```python
from build123d import *

# Parameters (mm, degrees)
BOSS_EXTRUDE1_DEPTH = 15
BOSS_EXTRUDE2_DEPTH = 20
SKETCH3_R           = 2.25
CUT_EXTRUDE1_DEPTH  = 15


with BuildPart() as part:
    # Sketch1 → Boss-Extrude1 (new, symmetric)
    with BuildSketch(Plane(origin=(0, 0, 0), x_dir=(1, 0, 0), z_dir=(0, 1, 0))):
        with BuildLine():
            Line((0, 0), (-27.5, 0))
            Line((-27.5, 0), (-22.5, -5))
            Line((-22.5, -5), (-44.5, -5))
            Line((-44.5, -5), (-44.5, 10))
            Line((-44.5, 10), (-35, 10))
            Line((-35, 10), (-35, 20))
            Line((-35, 20), (-25, 20))
            ThreePointArc((-25, 20), (-17.5, 12.5), (-10, 20))
            Line((-10, 20), (10, 20))
            ThreePointArc((10, 20), (17.5, 12.5), (25, 20))
            Line((25, 20), (35, 20))
            Line((35, 20), (35, 10))
            Line((35, 10), (44.5, 10))
            Line((44.5, 10), (44.5, -5))
            Line((44.5, -5), (22.5, -5))
            Line((22.5, -5), (27.5, 0))
            Line((27.5, 0), (0, 0))
        make_face()
    extrude(amount=BOSS_EXTRUDE1_DEPTH, both=True)

    # Sketch2 → Boss-Extrude2 (add, symmetric)
    with BuildSketch(Plane(origin=(0, 0, 0), x_dir=(1, 0, 0), z_dir=(0, 1, 0))):
        with BuildLine():
            Line((-30, 20), (-25, 20))
            ThreePointArc((-25, 20), (-17.5, 12.5), (-10, 20))
            Line((-10, 20), (5, 20))
            Line((5, 20), (10, 20))
            ThreePointArc((10, 20), (17.5, 12.5), (25, 20))
            Line((25, 20), (30, 20))
            ThreePointArc((30, 20), (26.338834765, 11.161165235), (17.5, 7.5))
            Line((17.5, 7.5), (7.664635512, 7.5))
            Line((7.664635512, 7.5), (7.664635512, 0))
            Line((7.664635512, 0), (-7.335364488, 0))
            Line((-7.335364488, 0), (-7.335364488, 7.5))
            Line((-7.335364488, 7.5), (-17.5, 7.5))
            ThreePointArc((-17.5, 7.5), (-26.338834765, 11.161165235), (-30, 20))
        make_face()
    extrude(amount=BOSS_EXTRUDE2_DEPTH, both=True)

    # Sketch3 → Cut-Extrude1 (cut)
    with BuildSketch(Plane(origin=(0, 0, -20), x_dir=(-1, 0, 0), z_dir=(0, 0, -1))):
        with Locations((0, 15)):
            Circle(SKETCH3_R)
        with Locations((-30, 7.5)):
            Circle(SKETCH3_R)
        with Locations((-30, -7.5)):
            Circle(SKETCH3_R)
        with Locations(Location((30, -7.5, 0), (0, 0, 180))):
            Circle(SKETCH3_R)
        with Locations(Location((30, 7.5, 0), (0, 0, 180))):
            Circle(SKETCH3_R)
        with Locations(Location((0, -15, 0), (0, 0, 180))):
            Circle(SKETCH3_R)
    extrude(amount=-CUT_EXTRUDE1_DEPTH, mode=Mode.SUBTRACT)


solid = part.part
```
Input: part model. Units: mm. Frame: model coordinates. A direction names the side the tool comes from. Give positions to 0.01 mm unless a question says otherwise; leave off trailing zeros. Order: outer loops, then holes, each group sorted by start corner. A loop starts at its lowest first (then second) coordinate and runs counter-clockwise, first axis right, second up. Notation, with made-up numbers: M 16.25,-39 L 58.25,-39 A30 ccw 58.25,-15 Z; hole C 69.5,-1.75 d4. An arc over 180 degrees is marked long. Return JSON: item names as keys, results as strings.
1) Section query D-D on z = -8.5. Output: boundary loops of the cut face in (x, y), and give its area (3 significant figures).
Taken from the geometry:
{"outline": "M -44.5,-15 L -22.4,-15 L -22.4,-20 L 22.4,-20 L 22.4,-15 L 44.5,-15 L 44.5,15 L 22.4,15 L 22.4,20 L -22.4,20 L -22.4,15 L -44.5,15 Z; hole C -30,-7.5 d4.5; hole C -30,7.5 d4.5; hole C 0,-15 d4.5; hole C 0,15 d4.5; hole C 30,-7.5 d4.5; hole C 30,7.5 d4.5", "area": "3,020 mm2"}
2) Access query for faces 1 (the face through (-35, 0, -15)), 2 (the face through (-12, -17, -7.5)), 3 (the face through (0, 15, -5)), 4 (the face through (13, 18, -7.5)). Directions: +Z, -Z, +X, -X, +Y, -Y. A direction counts if a zero-diameter tool reaches every point of the face in a straight line with its end or side. Return the directions, or none.
Taken from the geometry:
{"face 1": "-Z, -X, +Y, -Y", "face 2": "+Z, -X, -Y", "face 3": "-Z", "face 4": "+Z, +X, +Y"}
3) Section query B-B on z = -3.75. Output: boundary loops of the cut face in (x, y), and give its area (3 significant figures).
Taken from the geometry:
{"outline": "M -44.5,-15 L -7.34,-15 L -7.34,-20 L 7.66,-20 L 7.66,-15 L 44.5,-15 L 44.5,15 L 7.66,15 L 7.66,20 L -7.34,20 L -7.34,15 L -44.5,15 Z", "area": "2,820 mm2"}
4) Line query: L1, parallel to Y at x = -30, z = -9.5; L2, parallel to Y at x = 35, z = -3; L3, parallel to Z at x = -27, y = -11. Output: solid intervals per line, ascending. Write a range as [from, to].
Taken from the geometry:
{"L1": "y = [-15, -9.75], [-5.25, 5.25], [9.75, 15]", "L2": "y = [-15, 15]", "L3": "z = [-20, 0], [0.5, 5]"}
5) Section query A-A on y = 7.5. Output: boundary loops of the cut face in (x, z), and give its area (3 significant figures).
Taken from the geometry:
{"outline": "M -44.5,-10 L -35,-10 L -35,-20 L -32.25,-20 L -32.25,-5 L -27.75,-5 L -27.75,-20 L -25,-20 A7.5 cw -10,-20 L 10,-20 A7.5 cw 25,-20 L 27.75,-20 L 27.75,-5 L 32.25,-5 L 32.25,-20 L 35,-20 L 35,-10 L 44.5,-10 L 44.5,5 L 22.5,5 L 27.5,0 L -27.5,0 L -22.5,5 L -44.5,5 Z", "area": "1,470 mm2"}
6) Section query C-C on x = 38. Output: boundary loops of the cut face in (y, z), and give its area (3 significant figures).
Taken from the geometry:
{"outline": "M -15,-10 L 15,-10 L 15,5 L -15,5 Z", "area": "450 mm2"}
7) Mould query, pull axis Y, two halves, no side actions, for faces 5 (the face through (-12, 18, -7.5)), 6 (the face through (30, -15, -5)), 7 (the face through (30, 15, -5)), 8 (the face through (0, -15, -5)). Classes: released by +Y, released by -Y, zero draft, split by the parting line, or undercut.
Taken from the geometry:
{"face 5": "zero draft", "face 6": "released by -Y", "face 7": "released by +Y", "face 8": "undercut"}
8) Contact query for flat-ended pins moving along their axis: pin 1 (4 mm diameter, centred on y = -18.5, z = -4, fed in from -X); pin 2 (4 mm diameter, centred on x = -30, y = -7.5, fed in from -Z); pin 3 (2.5 mm diameter, centred on y = -16.5, z = -3, fed in from +X). Output: stop coordinate, or through.
Taken from the geometry:
{"pin 1": "stops at x = -7.34", "pin 2": "stops at z = -5", "pin 3": "stops at x = 7.66"}
